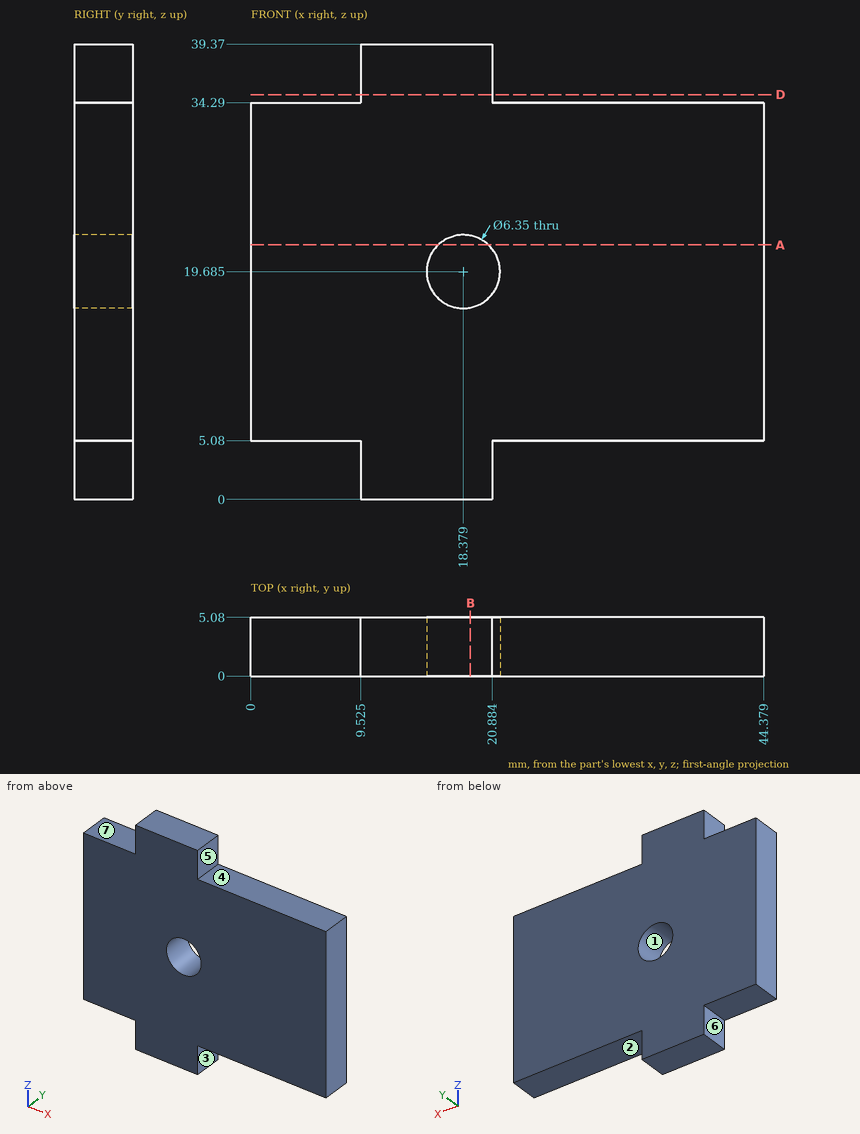
Print and shaded views of the part. All mm, measured from the part's lowest x, y and z. A direction names the side the tool comes from. Coordinates: 2 decimals unless noted, no trailing zeros. Write each loop counter-clockwise with the first axis right and the second up, starting at its lowest first coordinate (ties: lowest second). Pieces come first, ordered by that corner, then holes. Notation, with made-up numbers: (86.5, -34) -> (118.5, -34) arc R23 cw to (118.5, 4) -> close; hole circle Ø5 at (27, -38). An arc over 180 degrees is marked (long way). Use CSV: the item, a comma, the result in double quotes. Start each with the question number.
Q1. Cut at D-D, the plane z = 35. List the corners of the cut face in (x, y) (1 decimal).
Q2. Cut at A-A, the plane z = 22. List the corners of the cut face in (x, y).
Q3. 3-axis set-ups, long thin cutter, end or side, ignore diameter. For the marked faces 5, 6 and 7: which of +Z, -Z, +X, -X, +Y, -Y reach the whole face in a straight line?
Q4. Cut at B-B, the plane x = 19. List the corners of the cut face in (y, z), then the cut area to 3 significant figures.
Q5. Pull direction Z, two halves, no side cores. Call the marked faces 1, 2, 3 and 4: released by +Z, released by -Z, zero draft, split by the parting line, or undercut.
Q6. Flat gauge pins, fed straight in: pin 1 Ø2.5 at (x, y) = (5, 2) entering from +Z; pin 2 Ø1.5 at (y, z) = (1.5, 2.5) entering from +X. Where does each tip first touch, or does it go through?
Q7. Drill centre lines: probe 1 along Z at (x, y) = (29.5, 3.1); probe 2 along X at (y, z) = (4.15, 20); probe 3 along Z at (x, y) = (19.5, 0.8) (1 decimal). Where is each one in solid material? Low to high.
Checked values:
1,outline,"(9.5, 0) -> (20.9, 0) -> (20.9, 5.1) -> (9.5, 5.1) -> close"
2,outline,"(0, 0) -> (16.21, 0) -> (16.21, 5.08) -> (0, 5.08) -> close; (20.55, 0) -> (44.38, 0) -> (44.38, 5.08) -> (20.55, 5.08) -> close"
3,face 5,"+Z, +X, +Y, -Y"
3,face 6,"-Z, -X, +Y, -Y"
3,face 7,"+Z, -X, +Y, -Y"
4,outline,"(0, 0) -> (5.08, 0) -> (5.08, 16.57) -> (0, 16.57) -> close; (0, 22.8) -> (5.08, 22.8) -> (5.08, 39.37) -> (0, 39.37) -> close"
4,area,"168 mm²"
5,face 1,"undercut"
5,face 2,"released by -Z"
5,face 3,"zero draft"
5,face 4,"released by +Z"
6,pin 1,"stops at z = 34.29"
6,pin 2,"stops at x = 20.88"
7,probe 1,"z = 5.08 to 34.29"
7,probe 2,"x = 0 to 15.22, 21.54 to 44.38"
7,probe 3,"z = 0 to 16.7, 22.7 to 39.4"
